from build123d import *

# Parameters (mm, degrees)
SKETCH1_R           = 1.27
SKETCH1_W           = 59
SKETCH1_H           = 36
BOSS_EXTRUDE1_DEPTH = 1.6
SKETCH1_4_W         = 59
SKETCH1_4_H         = 36
BOSS_EXTRUDE2_DEPTH = 3.6
SKETCH2_W           = 22.9
SKETCH2_H           = 2.51
BOSS_EXTRUDE3_DEPTH = 10.66


with BuildPart() as part:
    # Sketch1 → Boss-Extrude1 (new body)
    # profile 1 of 2: a face of its own
    with BuildSketch(Plane.XY):
        with BuildLine():
            Line((0, 0), (0, -53.88))
            ThreePointArc((0, -53.88), (0.585786438, -55.294213562), (2, -55.88))
            Line((2, -55.88), (3.08, -55.88))
            ThreePointArc((3.08, -55.88), (4.494213562, -55.294213562), (5.08, -53.88))
            Line((5.08, -53.88), (5.08, -53.562))
            ThreePointArc((5.08, -53.562), (5.665786438, -52.147786438), (7.08, -51.562))
            Line((7.08, -51.562), (56.42, -51.562))
            ThreePointArc((56.42, -51.562), (57.834213562, -52.147786438), (58.42, -53.562))
            Line((58.42, -53.562), (58.42, -53.88))
            ThreePointArc((58.42, -53.88), (59.005786438, -55.294213562), (60.42, -55.88))
            Line((60.42, -55.88), (61.5, -55.88))
            ThreePointArc((61.5, -55.88), (62.914213562, -55.294213562), (63.5, -53.88))
            Line((63.5, -53.88), (63.5, 0))
            Line((63.5, 0), (0, 0))
        make_face()
        with Locations((2.54, -2.54)):
            Circle(SKETCH1_R, mode=Mode.SUBTRACT)
        with Locations((60.96, -2.54)):
            Circle(SKETCH1_R, mode=Mode.SUBTRACT)
        with Locations((60.96, -53.34)):
            Circle(SKETCH1_R, mode=Mode.SUBTRACT)
        with Locations((2.54, -53.34)):
            Circle(SKETCH1_R, mode=Mode.SUBTRACT)
        with Locations((31.75, -25.781)):
            Rectangle(SKETCH1_W, SKETCH1_H, mode=Mode.SUBTRACT)
    # profile 2 of 2: a face of its own
    with BuildSketch(Plane.XY):
        with Locations((31.75, -25.781)):
            Rectangle(SKETCH1_W, SKETCH1_H)
    extrude(amount=BOSS_EXTRUDE1_DEPTH)

    # Sketch1<4> → Boss-Extrude2 (add)
    with BuildSketch(Plane.XY):
        with Locations((31.75, -25.781)):
            Rectangle(SKETCH1_4_W, SKETCH1_4_H)
    extrude(amount=BOSS_EXTRUDE2_DEPTH)

    # Sketch2 → Boss-Extrude3 (add)
    with BuildSketch(Plane(origin=(0, 0, 0), x_dir=(-1, 0, 0), z_dir=(0, 0, -1))):
        with Locations((-31.75, -2.521379288)):
            Rectangle(SKETCH2_W, SKETCH2_H)
    extrude(amount=BOSS_EXTRUDE3_DEPTH)


solid = part.part
Work out the finished part from the listing and answer in its coordinate system (mm). A direction names the side the tool comes from. Coordinates: 2 decimals unless noted, no trailing zeros. Loops run counter-clockwise (first coordinate to the right, second up) from the corner with the lowest first, then second, coordinate; pieces in that order, holes last. Notation, with made-up numbers: M 28,-10 L 56,-10 A18 cw 56,3 Z; hole C -1.75,-30 d11. An arc over 180 degrees is marked long. Answer in a Markdown table with one row per item. Add a question column.
1. A tool of negligible diameter and unlimited length cuts with its end or side. For faces 1 (the flat face through (31, -43.781, 3)), 2 (the flat face through (31, -7.781, 3)), 3 (the cylindrical face through (57.819, -52.132, 0.789)), 4 (the flat face through (20.3, -3, -5)), from which of +Z, -Z, +X, -X, +Y, -Y can it reach the whole face along a straight path? Write none if from no direction.
2. The mould has two halves that part along X. Classify faces 5 (the cylindrical face through (58.99, -55.28, 0.79)), 6 (the flat face through (32, 0, 1)), 7 (the flat face through (0, -27, 1)): pulls with the +X half, pulls with the -X half, needs draft (parallel to the pull), parting line crosses it, or undercut.
3. Find section C-C, the plane y = -30. Write down the section's boundary in (x, z).
4. Flat-ended cylindrical pins translate along their axes: P1, Ø0.5, axis at x = 41, z = 0.5, coming from the -Y side; P2, Ø3, axis at x = 36.5, z = -5, coming from the -Y side; P3, Ø0.6, axis at x = 27.5, z = 2.5, coming from the -Y side; P4, Ø2, axis at x = 60.96, y = -2.54, coming from the +Z side. Find the tip coordinate at first contact, or state that the pin passes through.
5. Consider L1, parallel to Y at x = 60.96, z = 1.05; L2, parallel to X at y = -2.5, z = 1.5; L3, parallel to Y at x = 41, z = 2.75. Determine where each line is inside the solid, lowest interval first.
6. Find section D-D, the plane z = -4.75. Write down the section's boundary in (x, y).
7. Find section B-B, the plane x = 27. Write down the section's boundary in (y, z), then the cut area to 3 significant figures.
8. Find section A-A, the plane y = -2.54. Write down the section's boundary in (x, z).
Reported:
| question | item | result |
|---|---|---|
| 1 | face 1 | +Z, +X, -X, -Y |
| 1 | face 2 | +Z, +X, -X, +Y |
| 1 | face 3 | +Z, -Z, -Y |
| 1 | face 4 | -Z, -X, +Y, -Y |
| 2 | face 5 | undercut |
| 2 | face 6 | needs draft |
| 2 | face 7 | pulls with the -X half |
| 3 | outline | M 0,0 L 63.5,0 L 63.5,1.6 L 61.25,1.6 L 61.25,3.6 L 2.25,3.6 L 2.25,1.6 L 0,1.6 Z |
| 4 | P1 | stops at y = -51.56 |
| 4 | P2 | stops at y = -3.78 |
| 4 | P3 | stops at y = -43.78 |
| 4 | P4 | passes through |
| 5 | L1 | y = -55.88 to -54.61, -52.07 to -3.81, -1.27 to 0 |
| 5 | L2 | x = 0 to 1.27, 3.81 to 59.69, 62.23 to 63.5 |
| 5 | L3 | y = -43.78 to -7.78 |
| 6 | outline | M 20.3,-3.78 L 43.2,-3.78 L 43.2,-1.27 L 20.3,-1.27 Z |
| 7 | outline | M -51.56,0 L -3.78,0 L -3.78,-10.66 L -1.27,-10.66 L -1.27,0 L 0,0 L 0,1.6 L -7.78,1.6 L -7.78,3.6 L -43.78,3.6 L -43.78,1.6 L -51.56,1.6 Z |
| 7 | area | 181 mm^2 |
| 8 | outline | M 0,0 L 1.27,0 L 1.27,1.6 L 0,1.6 Z; M 3.81,0 L 20.3,0 L 20.3,-10.66 L 43.2,-10.66 L 43.2,0 L 59.69,0 L 59.69,1.6 L 3.81,1.6 Z; M 62.23,0 L 63.5,0 L 63.5,1.6 L 62.23,1.6 Z |
